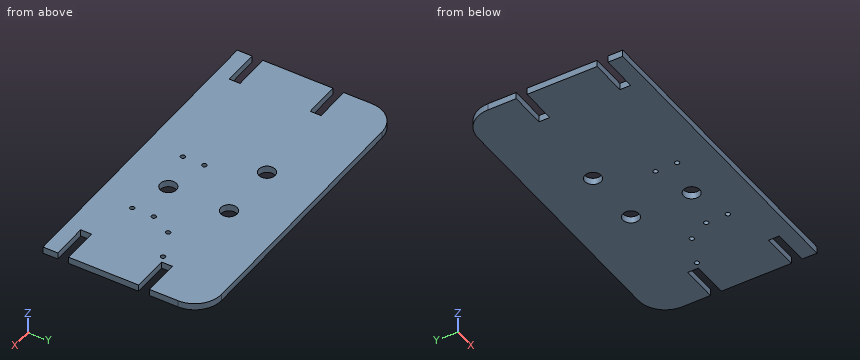
```python
from build123d import *

# Parameters (mm, degrees)
SKETCH1_W            = 230
SKETCH1_H            = 120
BOSS_EXTRUDE1_DEPTH  = 5
CUT_EXTRUDE1_REACH   = 131.808
SKETCH2_W            = 27
SKETCH2_H            = 8.000000001
CUT_EXTRUDE2_REACH   = 131.808
SKETCH3_R            = 6.025
M3_CLEARANCE_HOLE1_D = 3.4
FILLET1_R            = 20
CUT_EXTRUDE3_REACH   = 131.808
SKETCH7_R            = 1.7


with BuildPart() as part:
    # Sketch1 → Boss-Extrude1 (new body)
    with BuildSketch(Plane.XY):
        Rectangle(SKETCH1_W, SKETCH1_H)
    extrude(amount=BOSS_EXTRUDE1_DEPTH)

    # Sketch2 → Cut-Extrude1 (cut, up to next)
    with BuildSketch(Plane(origin=(0, 0, 0), x_dir=(-1, 0, 0), z_dir=(0, 0, -1)), mode=Mode.PRIVATE) as cut_extrude1_sk1:
        with Locations((101.5, 15.000000001)):
            Rectangle(SKETCH2_W, SKETCH2_H)
    cut_extrude1_tool1 = extrude(cut_extrude1_sk1.sketch, amount=-CUT_EXTRUDE1_REACH, mode=Mode.PRIVATE) & part.part
    # Sketch2 → Cut-Extrude1 (cut, up to next)
    with BuildSketch(Plane(origin=(0, 0, 0), x_dir=(-1, 0, 0), z_dir=(0, 0, -1)), mode=Mode.PRIVATE) as cut_extrude1_sk2:
        with Locations((101.5, -45.000000001)):
            Rectangle(SKETCH2_W, SKETCH2_H)
    cut_extrude1_tool2 = extrude(cut_extrude1_sk2.sketch, amount=-CUT_EXTRUDE1_REACH, mode=Mode.PRIVATE) & part.part
    # Sketch2 → Cut-Extrude1 (cut, up to next)
    with BuildSketch(Plane(origin=(0, 0, 0), x_dir=(-1, 0, 0), z_dir=(0, 0, -1)), mode=Mode.PRIVATE) as cut_extrude1_sk3:
        with Locations((-101.5, -45.000000001)):
            Rectangle(SKETCH2_W, SKETCH2_H)
    cut_extrude1_tool3 = extrude(cut_extrude1_sk3.sketch, amount=-CUT_EXTRUDE1_REACH, mode=Mode.PRIVATE) & part.part
    # Sketch2 → Cut-Extrude1 (cut, up to next)
    with BuildSketch(Plane(origin=(0, 0, 0), x_dir=(-1, 0, 0), z_dir=(0, 0, -1)), mode=Mode.PRIVATE) as cut_extrude1_sk4:
        with Locations((-101.5, 15.000000001)):
            Rectangle(SKETCH2_W, SKETCH2_H)
    cut_extrude1_tool4 = extrude(cut_extrude1_sk4.sketch, amount=-CUT_EXTRUDE1_REACH, mode=Mode.PRIVATE) & part.part
    add(cut_extrude1_tool1.solids().sort_by_distance((-101.5, 15, 0))[0], mode=Mode.SUBTRACT)
    add(cut_extrude1_tool2.solids().sort_by_distance((-101.5, -45, 0))[0], mode=Mode.SUBTRACT)
    add(cut_extrude1_tool3.solids().sort_by_distance((101.5, -45, 0))[0], mode=Mode.SUBTRACT)
    add(cut_extrude1_tool4.solids().sort_by_distance((101.5, 15, 0))[0], mode=Mode.SUBTRACT)

    # Sketch3 → Cut-Extrude2 (cut, up to next)
    with BuildSketch(Plane.XY.offset(5), mode=Mode.PRIVATE) as cut_extrude2_sk1:
        with Locations((22.5, 20)):
            Circle(SKETCH3_R)
    cut_extrude2_tool1 = extrude(cut_extrude2_sk1.sketch, amount=-CUT_EXTRUDE2_REACH, mode=Mode.PRIVATE) & part.part
    # Sketch3 → Cut-Extrude2 (cut, up to next)
    with BuildSketch(Plane.XY.offset(5), mode=Mode.PRIVATE) as cut_extrude2_sk2:
        with Locations((-22.5, 20)):
            Circle(SKETCH3_R)
    cut_extrude2_tool2 = extrude(cut_extrude2_sk2.sketch, amount=-CUT_EXTRUDE2_REACH, mode=Mode.PRIVATE) & part.part
    # Sketch3 → Cut-Extrude2 (cut, up to next)
    with BuildSketch(Plane.XY.offset(5), mode=Mode.PRIVATE) as cut_extrude2_sk3:
        with Locations((22.5, -25)):
            Circle(SKETCH3_R)
    cut_extrude2_tool3 = extrude(cut_extrude2_sk3.sketch, amount=-CUT_EXTRUDE2_REACH, mode=Mode.PRIVATE) & part.part
    add(cut_extrude2_tool1.solids().sort_by_distance((22.5, 20, 5))[0], mode=Mode.SUBTRACT)
    add(cut_extrude2_tool2.solids().sort_by_distance((-22.5, 20, 5))[0], mode=Mode.SUBTRACT)
    add(cut_extrude2_tool3.solids().sort_by_distance((22.5, -25, 5))[0], mode=Mode.SUBTRACT)

    # M3 Clearance Hole1 (through all)
    with Locations(Plane(origin=(-7.5, -17, 5), x_dir=(1, 0, 0), z_dir=(0, 0, 1))):
        with Locations((0, 0), (60, 0), (60, -16), (0, -16)):
            Hole(M3_CLEARANCE_HOLE1_D / 2)

    # Fillet1
    fillet1_edges = [part.edges().sort_by_distance(p)[0] for p in [
        (-115, 60, 2.5),
        (115, 60, 2.5),
    ]]
    fillet(fillet1_edges, radius=FILLET1_R)

    # Sketch7 → Cut-Extrude3 (cut, up to next)
    with BuildSketch(Plane.XY.offset(5), mode=Mode.PRIVATE) as cut_extrude3_sk1:
        with Locations((61, -1)):
            Circle(SKETCH7_R)
    cut_extrude3_tool1 = extrude(cut_extrude3_sk1.sketch, amount=-CUT_EXTRUDE3_REACH, mode=Mode.PRIVATE) & part.part
    # Sketch7 → Cut-Extrude3 (cut, up to next)
    with BuildSketch(Plane.XY.offset(5), mode=Mode.PRIVATE) as cut_extrude3_sk2:
        with Locations((83, 9)):
            Circle(SKETCH7_R)
    cut_extrude3_tool2 = extrude(cut_extrude3_sk2.sketch, amount=-CUT_EXTRUDE3_REACH, mode=Mode.PRIVATE) & part.part
    add(cut_extrude3_tool1.solids().sort_by_distance((61, -1, 5))[0], mode=Mode.SUBTRACT)
    add(cut_extrude3_tool2.solids().sort_by_distance((83, 9, 5))[0], mode=Mode.SUBTRACT)


solid = part.part
```
CAD build for the part. Positions are in the model's coordinates, mm. Coordinates: 2 decimals unless noted, no trailing zeros. Order: outer loops, then holes, each group sorted by start corner. A loop starts at its lowest first (then second) coordinate and runs counter-clockwise, first axis right, second up. Notation, with made-up numbers: (70.25, 64.5) - (117.25, 64.5) arc R10 cw to (117.25, 74.5) - close; hole circle Ø3 at (81.5, 47). An arc over 180 degrees is marked (long way). Use a Markdown table: item, result. Add a question column.
(1) Saw through at B-B (z = 3.4). Count the separate pieces of the cut face and the enclosed holes in it, then the cut area to 3 significant figures.
(2) Saw through at A-A (x = 92). Give the cut face in (y, z).
(3) Drill centre lines: line 1 along Y through (x, z) = (22, 3.05); line 2 along Y through (x, z) = (92, 2.2); line 3 along Y through (x, z) = (83, 2.2). Where is each one in solid material? Low to high. Write a range as [from, to].
(4) Flat gauge pins, fed straight in: pin 1 (2.5 mm diameter, centred on x = 98, z = 1.5, fed in from +Y); pin 2 (5.5 mm diameter, centred on x = -7.5, y = -33, fed in from -Z); pin 3 (1 mm diameter, centred on y = 42.5, z = 2, fed in from +X). Where does each tip first touch, or does it go through?
Solved:
| question | item | result |
|---|---|---|
| 1 | separate pieces | 1 |
| 1 | enclosed holes | 9 |
| 1 | area | 26,200 mm² |
| 2 | outline | (-60, 0) - (-49, 0) - (-49, 5) - (-60, 5) - close; (-41, 0) - (11, 0) - (11, 5) - (-41, 5) - close; (19, 0) - (60, 0) - (60, 5) - (19, 5) - close |
| 3 | line 1 | y = [-60, -31], [-19, 14], [26, 60] |
| 3 | line 2 | y = [-60, -49], [-41, 11], [19, 60] |
| 3 | line 3 | y = [-60, 7.3], [10.7, 60] |
| 4 | pin 1 | stops at y = 59.92 |
| 4 | pin 2 | stops at z = 0 |
| 4 | pin 3 | stops at x = 114.9 |
